Design review of the part built by this model. Coordinates are the model's own, in mm. Face numbers are marked on the shaded views. A direction names the side the tool comes from. Round coordinates to 2 decimals unless told otherwise and drop trailing zeros. Loops run counter-clockwise (first coordinate to the right, second up) from the corner with the lowest first, then second, coordinate; pieces in that order, holes last. Notation, with made-up numbers: M 34.25,30 L 89.25,30 A17 ccw 89.25,60 Z; hole C 0,0 d11. An arc over 180 degrees is marked long. Use a Markdown table: item, result.
from build123d import *

# Parameters (mm, degrees)
BOSS_EXTRUDE1_DEPTH  = 9
CUT_EXTRUDE1_DEPTH   = 79.339006887
FILLET1_R            = 6
FILLET4_R            = 3
FILLET5_R            = 10
FILLET1_OF_MIRROR2_R = 6
FILLET4_OF_MIRROR2_R = 3
FILLET5_OF_MIRROR2_R = 10
CUT_EXTRUDE2_DEPTH   = 2
SKETCH4_W            = 7.3
SKETCH4_H            = 3.5
CUT_EXTRUDE3_DEPTH   = 79.134499565
CUT_EXTRUDE4_DEPTH   = 89.260976804


with BuildPart() as part:
    # Sketch1 → Boss-Extrude1 (new body)
    with BuildSketch(Plane.XY):
        with BuildLine():
            Line((-70, 16.58258549), (-70, 2.58258549))
            Line((-70, 2.58258549), (-65, -0.035347018))
            ThreePointArc((-65, -0.035347018), (-62.639321295, -11.428715409), (-59.057390955, -22.499009997))
            ThreePointArc((-59.057390955, -22.499009997), (-50.858075368, -30.911196539), (-39.524366721, -34))
            Line((-39.524366721, -34), (-29.119439011, -34))
            ThreePointArc((-29.119439011, -34), (-16.364659062, -29.873537236), (-8.443933007, -19.058075838))
            ThreePointArc((-8.443933007, -19.058075838), (-5.792248942, -9.629238804), (-4, 0))
            Line((-4, 0), (0, 0))
            Line((0, 0), (0, 19))
            Line((0, 19), (-62, 19))
            Line((-62, 19), (-70, 16.58258549))
        make_face()
    boss_extrude1 = extrude(amount=BOSS_EXTRUDE1_DEPTH)

    # Sketch2 → Cut-Extrude1 (cut, through all)
    with BuildSketch(Plane.XY.offset(9)):
        with BuildLine():
            Line((-39.524366721, -29), (-29.119439011, -29))
            ThreePointArc((-29.119439011, -29), (-19.293350153, -25.821035725), (-13.191343035, -17.488968441))
            ThreePointArc((-13.191343035, -17.488968441), (-10.661621804, -8.493805879), (-8.951806424, 0.692541077))
            ThreePointArc((-8.951806424, 0.692541077), (-8.83111114, 2.375291538), (-8.93749946, 4.05900707))
            ThreePointArc((-8.93749946, 4.05900707), (-33.987475013, 7.999161751), (-59.288689209, 6.303681198))
            ThreePointArc((-59.288689209, 6.303681198), (-60.075532666, 3.563074376), (-60.056140486, 0.711816353))
            ThreePointArc((-60.056140486, 0.711816353), (-57.852345066, -9.972645379), (-54.521869403, -20.361214511))
            ThreePointArc((-54.521869403, -20.361214511), (-48.178176596, -26.685865227), (-39.524366721, -29))
        make_face()
    cut_extrude1 = extrude(amount=-CUT_EXTRUDE1_DEPTH, mode=Mode.SUBTRACT)

    # Fillet1
    fillet1_edges = [part.edges().sort_by_distance(p)[0] for p in [
        (-8.93749946, 4.05900707, 4.5),
        (-59.288689209, 6.303681198, 4.5),
    ]]
    fillet(fillet1_edges, radius=FILLET1_R)

    # Fillet4
    fillet4_edges = [part.edges().sort_by_distance(p)[0] for p in [
        (-4, 0, 4.5),
    ]]
    fillet(fillet4_edges, radius=FILLET4_R)

    # Fillet5
    fillet5_edges = [part.edges().sort_by_distance(p)[0] for p in [
        (-65, -0.035347018, 4.5),
        (-62, 19, 4.5),
    ]]
    fillet(fillet5_edges, radius=FILLET5_R)

    # Mirror2: Boss-Extrude1, Cut-Extrude1 across plane
    add(boss_extrude1.mirror(Plane(origin=(0, 19, 9), x_dir=(0, 0, 1), z_dir=(1, 0, 0))))
    add(cut_extrude1.mirror(Plane(origin=(0, 19, 9), x_dir=(0, 0, 1), z_dir=(1, 0, 0))), mode=Mode.SUBTRACT)

    # Fillet1 of Mirror2
    fillet1_of_mirror2_edges = [part.edges().sort_by_distance(p)[0] for p in [
        (8.93749946, 4.05900707, 4.5),
        (59.288689209, 6.303681198, 4.5),
    ]]
    fillet(fillet1_of_mirror2_edges, radius=FILLET1_OF_MIRROR2_R)

    # Fillet4 of Mirror2
    fillet4_of_mirror2_edges = [part.edges().sort_by_distance(p)[0] for p in [
        (4, 0, 4.5),
    ]]
    fillet(fillet4_of_mirror2_edges, radius=FILLET4_OF_MIRROR2_R)

    # Fillet5 of Mirror2
    fillet5_of_mirror2_edges = [part.edges().sort_by_distance(p)[0] for p in [
        (65, -0.035347018, 4.5),
        (62, 19, 4.5),
    ]]
    fillet(fillet5_of_mirror2_edges, radius=FILLET5_OF_MIRROR2_R)

    # Sketch3 → Cut-Extrude2 (cut)
    with BuildSketch(Plane.XY.offset(9)):
        Polygon((-68.579000582, 15.967320332), (-61.852211578, 18), (61.852211578, 18), (68.579000582, 15.967320332), (68.579000582, 2.967348727), (66.731457293, 2), (61.632252323, 2), (57.126911514, 9.5), (18.95111491, 9.5), (4.382114171, 2), (-4.382114171, 2), (-18.95111491, 9.5), (-57.126911514, 9.5), (-61.632252323, 2), (-66.731457293, 2), (-68.579000582, 2.967348727), align=None)
    extrude(amount=-CUT_EXTRUDE2_DEPTH, mode=Mode.SUBTRACT)

    # Sketch4 → Cut-Extrude3 (cut, through all)
    with BuildSketch(Plane.XY.offset(7)):
        with Locations((0, 14)):
            Rectangle(SKETCH4_W, SKETCH4_H)
        with Locations((0, 6.5)):
            Rectangle(SKETCH4_W, SKETCH4_H)
    extrude(amount=-CUT_EXTRUDE3_DEPTH, mode=Mode.SUBTRACT)

    # Sketch5 → Cut-Extrude4 (cut, through all)
    with BuildSketch(Plane(origin=(0, 19, 0), x_dir=(1, 0, 0), z_dir=(0, 1, 0))):
        with BuildLine():
            Line((-70, 0), (70, 0))
            ThreePointArc((70, 0), (38.581705318, -3.529487002), (7, -5))
            ThreePointArc((7, -5), (0, -6.753122833), (-7, -5))
            ThreePointArc((-7, -5), (-38.581705318, -3.529487002), (-70, 0))
        make_face()
    extrude(amount=-CUT_EXTRUDE4_DEPTH, mode=Mode.SUBTRACT)


solid = part.part
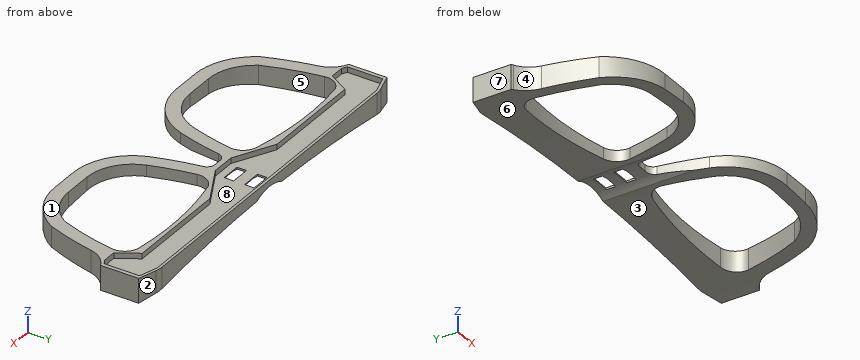
1. Machinability: for the marked faces 4, 5, 6, 7 and 8, which of the approach directions +Z, -Z, +X, -X, +Y, -Y give a long, thin tool a straight path to every point of the face, cutting with its end or side? Answer none if there is none.
Check values:
| item | result |
|---|---|
| face 4 | +Z, -Z, -X, -Y |
| face 5 | +Z, -Z |
| face 6 | -Z, +Y, -Y |
| face 7 | +Z, -Z, -X, +Y, -Y |
| face 8 | +Z |
2. Take a section at C-C on x = 16. Give the boundary of the cut face in (y, z).
Check values:
| item | result |
|---|---|
| outline | M -29.6,4.79 L -22.68,4.79 L -22.68,9 L -29.6,9 Z; M 5.75,4.79 L 19,4.79 L 19,9 L 18,9 L 18,7 L 7.98,7 L 7.98,9 L 5.75,9 Z |
3. Wall thickness on line 1 along X through (y, z) = (-3.5, 5.25); line 2 along Y through (x, z) = (-44, 7.5); line 3 along X through (y, z) = (-24.5, 8.5): over which ranges is each line inside the solid? List them lowest first. Write a range as from..to.
Check values:
| item | result |
|---|---|
| line 1 | x = -64.5..-59.33, -9.63..-6.51, 6.51..9.63, 59.33..64.5 |
| line 2 | y = -33.55..-28.41, 8.01..9.5, 18..19 |
| line 3 | x = -57.8..-51.18, -17.69..-11.13, 11.13..17.69, 51.18..57.8 |
4. Take a section at A-A on x = 48. Give the boundary of the cut face in (y, z).
Check values:
| item | result |
|---|---|
| outline | M -32.33,2.69 L -26.79,2.69 L -26.79,9 L -32.33,9 Z; M 7.76,2.69 L 19,2.69 L 19,9 L 18,9 L 18,7 L 9.5,7 L 9.5,9 L 7.76,9 Z |
5. The part is to be moulded in two halves that separate along X. For the marked faces 1, 2 and 3, say which applies: pulls with the +X half, pulls with the -X half, needs draft (parallel to the pull), parting line crosses it, or undercut.
Check values:
| item | result |
|---|---|
| face 1 | needs draft |
| face 2 | pulls with the +X half |
| face 3 | undercut |
6. Take a section at B-B on y = -11. Give the boundary of the cut face in (x, z), and give its area (3 significant figures).
Check values:
| item | result |
|---|---|
| outline | M -62.75,1 A483.95 cw -57.58,1.64 L -57.58,9 L -62.75,9 Z; M -11.28,4.92 A483.95 cw -7,5 A14.85 cw -6.12,5.43 L -6.12,9 L -11.28,9 Z; M 6.12,5.43 A14.85 cw 7,5 A483.95 cw 11.28,4.92 L 11.28,9 L 6.12,9 Z; M 57.58,1.64 A483.95 cw 62.75,1 L 62.75,9 L 57.58,9 Z |
| area | 121 mm² |
7. Insertion check: pin 1 (0.6 mm diameter, centred on x = 1.5, z = 6.5, fed in from -Y); pin 2 (5 mm diameter, centred on x = -0.5, y = 1.5, fed in from -Z); pin 3 (3 mm diameter, centred on x = 24.5, z = 5.5, fed in from -Y). Each pin has a flat end and moves straight along its axis. Give the tip position at first contact, or say it passes through.
Check values:
| item | result |
|---|---|
| pin 1 | stops at y = -0.02 |
| pin 2 | stops at z = 6.45 |
| pin 3 | stops at y = -33.78 |
8. Take a section at D-D on y = -24. Give the boundary of the cut face in (x, z).
Check values:
| item | result |
|---|---|
| outline | M -58.15,1.58 A483.95 cw -51.71,2.31 L -51.71,9 L -58.15,9 Z; M -17.17,4.75 A483.95 cw -10.8,4.93 L -10.8,9 L -17.17,9 Z; M 10.8,4.93 A483.95 cw 17.17,4.75 L 17.17,9 L 10.8,9 Z; M 51.71,2.31 A483.95 cw 58.15,1.58 L 58.15,9 L 51.71,9 Z |
